```python
from build123d import *

# Parameters (mm, degrees)
BOSS_EXTRU_1_DEPTH      = 10
ESQUISSE2_R             = 1
ENL_V_MAT_EXTRU_1_DEPTH = 10
ENL_V_MAT_EXTRU_3_DEPTH = 20


with BuildPart() as part:
    # Esquisse1 → Boss.-Extru.1 (new body)
    with BuildSketch(Plane.XY):
        Polygon((-108.571776559, 155.097150605), (-117.644392871, 150.891483803), (-107.130225868, 128.209943022), (-104.408440974, 129.471643062), (-109.455241136, 140.358782637), (-105.826194611, 142.041049358), (-100.779394449, 131.153909783), (-98.057609555, 132.415609823), align=None)
    extrude(amount=BOSS_EXTRU_1_DEPTH)

    # Esquisse2 → Enlèv. mat.-Extru.1 (cut)
    with BuildSketch(Plane(origin=(-39.261124148, -18.199734313, 0), x_dir=(0, 0, 1), z_dir=(-0.9072616312569987, -0.4205666801458358, 0))):
        with BuildLine():
            Line((2.5, 186.375365486), (0, 186.375365486))
            Line((0, 186.375365486), (0, 176.375365486))
            add(Edge.make_bspline(
                [(2.5, 186.375365486), (2.488696379, 181.391976925), (0, 176.375365486)],
                knots=[0, 0, 0, 1, 1, 1], degree=2))
        make_face()
        with BuildLine():
            Line((10, 186.375365486), (2.5, 186.375365486))
            add(Edge.make_bspline(
                [(10, 176.375365486), (9.306148512, 186.375365486), (2.5, 186.375365486)],
                knots=[0, 0, 0, 1, 1, 1], degree=2))
            Line((10, 176.375365486), (10, 186.375365486))
        make_face()
        with BuildLine():
            ThreePointArc((5, 161.375365486), (1.464466094, 162.83983158), (0, 166.375365486))
            Line((0, 166.375365486), (0, 161.375365486))
            Line((0, 161.375365486), (5, 161.375365486))
        make_face()
        with BuildLine():
            Line((10, 161.375365486), (10, 166.375365486))
            ThreePointArc((10, 166.375365486), (8.535533906, 162.83983158), (5, 161.375365486))
            Line((5, 161.375365486), (10, 161.375365486))
        make_face()
        with Locations(Location((5, 166.375365486, 0), (0, 0, 270))):
            Circle(ESQUISSE2_R)
    extrude(amount=-ENL_V_MAT_EXTRU_1_DEPTH, mode=Mode.SUBTRACT)

    # Esquisse4 → Enlèv. mat.-Extru.3 (cut)
    with BuildSketch(Plane(origin=(0, 0, 0), x_dir=(-1, 0, 0), z_dir=(0, 0, -1))):
        with BuildLine():
            Line((113.108084486, 152.99431731), (108.571776559, 155.097150605))
            Line((108.571776559, 155.097150605), (106.468943158, 150.560842448))
            ThreePointArc((106.468943158, 150.560842448), (109.284524694, 153.15259102), (113.108084486, 152.99431731))
        make_face()
        with BuildLine():
            Line((117.644392871, 150.891483803), (113.108084486, 152.99431731))
            ThreePointArc((113.108084486, 152.99431731), (115.699833287, 150.178735668), (115.541559471, 146.355175647))
            Line((115.541559471, 146.355175647), (117.644392871, 150.891483803))
        make_face()
    extrude(amount=-ENL_V_MAT_EXTRU_3_DEPTH, mode=Mode.SUBTRACT)


solid = part.part
```
Design review of the part built by this model. Coordinates are the model's own, in mm. A direction names the side the tool comes from. Coordinates: 2 decimals unless noted, no trailing zeros. Write each loop counter-clockwise with the first axis right and the second up, starting at its lowest first coordinate (ties: lowest second). Pieces come first, ordered by that corner, then holes.
1) Insertion check: pin 1 (2 mm diameter, centred on y = 143, z = 2.5, fed in from -X); pin 2 (4 mm diameter, centred on y = 140, z = 7.5, fed in from -X); pin 3 (3 mm diameter, centred on x = -110, y = 148, fed in from -Z). Each pin has a flat end and moves straight along its axis. Give the tip position at first contact, or say it passes through.
2) Mouldability with a two-part tool opening along X and no side actions: class faces 1 (the cylindrical face through (-115.917, 149.391, 4.618)), 2 (the cylindrical face through (-107.5, 132.5, 5.3)), 3 (the flat face through (-102.204, 141.361, 4.93)), 4 (the cylindrical face through (-101.139, 135.447, 5.3)) as +X half, -X half, draft (parallel to the pull), parting line (faces both ways), or undercut.
3) Machinability: for faces 5 (the flat face through (-107.46, 136.05, 4.93)), 6 (the flat face through (-111.395, 137.41, 4.93)), which of the approach directions +Z, -Z, +X, -X, +Y, -Y give a long, thin tool a straight path to every point of the face, cutting with its end or side? Answer none if there is none.
4) Add section B-B (x = -107.5). State how many separate pieces and enclosed holes the cut face has, plus the area to 3 significant figures.
5) Add section A-A (y = 140). Write out the cut boundary in (x, z), plus the area to 3 significant figures.
6) To check wall thickness, follow L1, parallel to X at y = 137.5, z = 8.75; L2, parallel to X at y = 141.5, z = 4.75; L3, parallel to Y at x = -108.75, z = 7.5. State the ranges of each line that lie inside material, in increasing order.
Check result:
1. pin 1: stops at x = -114.45
1. pin 2: stops at x = -113.52
1. pin 3: stops at z = 1.15
2. face 1: -X half
2. face 2: undercut
2. face 3: +X half
2. face 4: undercut
3. face 5: +Z, -Z
3. face 6: +Z, -Z, -X, -Y
4. separate pieces: 2
4. enclosed holes: 1
4. area: 155 mm2
5. outline: (-112.6, 0) - (-109.29, 0) - (-109.29, 10) - (-112.6, 10) - close; (-104.88, 0) - (-101.57, 0) - (-101.57, 10) - (-104.88, 10) - close
5. area: 66.1 mm2
6. L1: x = -111.44 to -108.13, -103.72 to -100.41
6. L2: x = -113.29 to -106.99, -105.58 to -102.27
6. L3: y = 131.7 to 138.84, 140.69 to 152.64
